from build123d import *

# Parameters (mm, degrees)
SALIENTE_EXTRUIR1_DEPTH = 55
CORTAR_EXTRUIR3_DEPTH   = 113.026782512
CORTAR_EXTRUIR4_DEPTH   = 116
CROQUIS6_R              = 1.6
CORTAR_EXTRUIR5_DEPTH   = 20
CORTAR_EXTRUIR6_START   = -10
CORTAR_EXTRUIR6_DEPTH   = 3
CROQUIS8_R              = 2.1
CORTAR_EXTRUIR8_DEPTH   = 116
MATRIZL1_COUNT          = 8
MATRIZL1_PITCH          = 10
CHAFL_N1_SIZE           = 1
CROQUIS9_R              = 2.1
CORTAR_EXTRUIR11_DEPTH  = 130.421791055
MATRIZL2_COUNT          = 6
MATRIZL2_PITCH          = 10


with BuildPart() as part:
    # Croquis1 → Saliente-Extruir1 (new body)
    with BuildSketch(Plane.XY):
        Polygon((15, -6.213203436), (15, 6.213203436), (6.213203436, 15), (-6.213203436, 15), (-15, 6.213203436), (-15, -6.213203436), (-6.213203436, -15), (6.213203436, -15), align=None)
    saliente_extruir1 = extrude(amount=SALIENTE_EXTRUIR1_DEPTH)

    # Simetría1: Saliente-Extruir1 across plane
    add(saliente_extruir1.mirror(Plane.XY.offset(55)))

    # Croquis4 → Cortar-Extruir3 (cut, through all)
    with BuildSketch(Plane(origin=(0, 0, 0), x_dir=(-1, 0, 0), z_dir=(0, 0, -1))):
        Polygon((-5.773502692, 0), (-2.886751346, -5), (2.886751346, -5), (5.773502692, 0), (2.886751346, 5), (-2.886751346, 5), align=None)
    extrude(amount=-CORTAR_EXTRUIR3_DEPTH, mode=Mode.SUBTRACT)

    # Croquis5 → Cortar-Extruir4 (cut, through all)
    with BuildSketch(Plane.XZ.offset(15)):
        Polygon((-6.213203436, 110), (-6.213203436, 78.298736304), (-15, 40.569524353), (-15, 110), align=None)
    extrude(amount=-CORTAR_EXTRUIR4_DEPTH, mode=Mode.SUBTRACT)

    # Croquis6 → Cortar-Extruir5 (cut)
    with BuildSketch(Plane.XY.offset(110)):
        with Locations((0, 11)):
            Circle(CROQUIS6_R)
        with Locations((7.778174593, 7.778174593)):
            Circle(CROQUIS6_R)
        with Locations((11, 0)):
            Circle(CROQUIS6_R)
        with Locations((7.778174593, -7.778174593)):
            Circle(CROQUIS6_R)
        with Locations((0, -11)):
            Circle(CROQUIS6_R)
    extrude(amount=-CORTAR_EXTRUIR5_DEPTH, mode=Mode.SUBTRACT)

    # Croquis7 → Cortar-Extruir6 (cut)
    with BuildSketch(Plane.XY.offset(110).offset(CORTAR_EXTRUIR6_START)):
        Polygon((-2.75, 12.58771324), (-2.75, 18.463203436), (2.75, 23.963203436), (2.75, 12.58771324), (2.75, 9.41228676), (0, 7.824573519), (-2.75, 9.41228676), align=None)
        Polygon((6.956313744, 10.84540104), (11.110912703, 15), (18.889087297, 15), (10.84540104, 6.956313744), (8.600035443, 4.710948146), (5.532808996, 5.532808996), (4.710948146, 8.600035443), align=None)
        Polygon((12.58771324, 2.75), (18.463203436, 2.75), (23.963203436, -2.75), (12.58771324, -2.75), (9.41228676, -2.75), (7.824573519, 0), (9.41228676, 2.75), align=None)
        Polygon((10.84540104, -6.956313744), (15, -11.110912703), (15, -18.889087297), (6.956313744, -10.84540104), (4.710948146, -8.600035443), (5.532808996, -5.532808996), (8.600035443, -4.710948146), align=None)
        Polygon((2.75, -12.58771324), (2.75, -18.463203436), (-2.75, -23.963203436), (-2.75, -12.58771324), (-2.75, -9.41228676), (0, -7.824573519), (2.75, -9.41228676), align=None)
    extrude(amount=-CORTAR_EXTRUIR6_DEPTH, mode=Mode.SUBTRACT)

    # Croquis8 → Cortar-Extruir8 (cut, through all)
    with BuildSketch(Plane.XZ.offset(15)):
        with Locations((0, 5)):
            Circle(CROQUIS8_R)
    cortar_extruir8 = extrude(amount=-CORTAR_EXTRUIR8_DEPTH, mode=Mode.SUBTRACT)

    # MatrizL1: Cortar-Extruir8 ×8
    with Locations(*[(0, 0, i * MATRIZL1_PITCH) for i in range(1, MATRIZL1_COUNT)]):
        add(cortar_extruir8, mode=Mode.SUBTRACT)

    # Chaflán1
    # the kernel refuses this chamfer: 1 mm, written as the material it takes off along each edge
    with BuildSketch(Plane(origin=(-6.213203436, -15, 112.571682988), x_dir=(0.9996219169112968, -0.027495876610585623, 0), z_dir=(0, 0, -1))) as chafl_n1_piece_1_section:
        Polygon((CHAFL_N1_SIZE * 0.999621916911, -CHAFL_N1_SIZE * 0.0274958766106), (-CHAFL_N1_SIZE * 0.0274958766106, -CHAFL_N1_SIZE * 0.999621916911), (0, 0), align=None)
    chafl_n1_piece_1 = extrude(amount=34.272946684, mode=Mode.PRIVATE)
    chafl_n1_piece_1 = split(chafl_n1_piece_1, bisect_by=Plane(origin=(-2.540552648, -14.662726337, 94.068558556), z_dir=(-0.9739364396780411, 0, 0.22682110013678505)), keep=Keep.TOP, mode=Mode.PRIVATE)
    add(chafl_n1_piece_1, mode=Mode.SUBTRACT)
    with BuildSketch(Plane(origin=(-6.213203436, 15, 78.298736304), x_dir=(-0.027495876610583055, -0.9996219169112968, 0), z_dir=(0, 0, 1))) as chafl_n1_piece_2_section:
        Polygon((CHAFL_N1_SIZE * 0.999621916911, CHAFL_N1_SIZE * 0.0274958766106), (-CHAFL_N1_SIZE * 0.0274958766106, CHAFL_N1_SIZE * 0.999621916911), (0, 0), align=None)
    chafl_n1_piece_2 = extrude(amount=34.272946684, mode=Mode.PRIVATE)
    chafl_n1_piece_2 = split(chafl_n1_piece_2, bisect_by=Plane(origin=(-2.540552648, 14.662726337, 94.068558556), z_dir=(-0.9739364396780411, 0, 0.22682110013678505)), keep=Keep.TOP, mode=Mode.PRIVATE)
    add(chafl_n1_piece_2, mode=Mode.SUBTRACT)
    with BuildSketch(Plane(origin=(-6.213203436, -17.571682988, 110), x_dir=(0.999621916911297, 0, 0.027495876610582174), z_dir=(0, 1, 0))) as chafl_n1_piece_3:
        Polygon((CHAFL_N1_SIZE * 0.999621916911, CHAFL_N1_SIZE * 0.0274958766106), (-CHAFL_N1_SIZE * 0.0274958766106, CHAFL_N1_SIZE * 0.999621916911), (0, 0), align=None)
    extrude(amount=35.143365976, mode=Mode.SUBTRACT)

    # Croquis9 → Cortar-Extruir11 (cut, through all)
    with BuildSketch(Plane(origin=(15, 0, -15), x_dir=(0, 0, -1), z_dir=(-1, 0, 0))):
        with Locations((-25, 0)):
            Circle(CROQUIS9_R)
    cortar_extruir11 = extrude(amount=CORTAR_EXTRUIR11_DEPTH, mode=Mode.SUBTRACT)

    # MatrizL2: Cortar-Extruir11 ×6
    with Locations(*[(0, 0, i * MATRIZL2_PITCH) for i in range(1, MATRIZL2_COUNT)]):
        add(cortar_extruir11, mode=Mode.SUBTRACT)


solid = part.part
Build history of the part. All positions in model axes, mm. A direction names the side the tool comes from. Coordinates: 2 decimals unless noted, no trailing zeros. Order: outer loops, then holes, each group sorted by start corner. A loop starts at its lowest first (then second) coordinate and runs counter-clockwise, first axis right, second up. Notation, with made-up numbers: (81, 61.25) - (105, 61.25) arc R21 ccw to (105, 78.25) - close; hole circle Ø2 at (16.5, 59.25). An arc over 180 degrees is marked (long way). Put each result on its own line as item: value.
1. Tool access for faces 5 (the face through (13, 0, 100)), 6 (the face through (7.57, 9.365, 93.549)), 7 (the face through (-2.75, 12, 99)), 8 (the face through (0, -13, 97)), 9 (the face through (7.04, -5.13, 98.52)): list every direction of +Z, -Z, +X, -X, +Y, -Y with a clear straight run to the whole face (end or side of a thin tool).
Answer sheet:
face 5: +X
face 6: +Z
face 7: +Y
face 8: -Y
face 9: none
2. Pull direction Z, two halves, no side cores. Call faces 1 (the face through (-6.213, 0, 94)), 2 (the face through (10, 9, 97)), 3 (the face through (8.63, -1.394, 98.521)), 4 (the face through (7, 0, 110)): pulls with the +Z half, pulls with the -Z half, needs draft (parallel to the pull), parting line crosses it, or undercut.
Answer sheet:
face 1: needs draft
face 2: undercut
face 3: undercut
face 4: pulls with the +Z half
3. Saw through at A-A (z = 35). Write the cut outline in (x, y).
Answer sheet:
outline: (-15, -6.21) - (-6.21, -15) - (-2.1, -15) - (-2.1, -5) - (-2.89, -5) - (-5.77, 0) - (-2.89, 5) - (-2.1, 5) - (-2.1, 15) - (-6.21, 15) - (-15, 6.21) - close; (2.1, -15) - (6.21, -15) - (15, -6.21) - (15, 6.21) - (6.21, 15) - (2.1, 15) - (2.1, 5) - (2.89, 5) - (5.77, 0) - (2.89, -5) - (2.1, -5) - close
4. Saw through at B-B (z = 10). Write the cut outline in (x, y), and give its area (3 significant figures).
Answer sheet:
outline: (-15, -6.21) - (-6.21, -15) - (6.21, -15) - (15, -6.21) - (15, -2.1) - (4.56, -2.1) - (2.89, -5) - (-2.89, -5) - (-4.56, -2.1) - (-15, -2.1) - close; (-15, 2.1) - (-4.56, 2.1) - (-2.89, 5) - (2.89, 5) - (4.56, 2.1) - (15, 2.1) - (15, 6.21) - (6.21, 15) - (-6.21, 15) - (-15, 6.21) - close
area: 576 mm^2
5. Probe line 1 along Y through (x, z) = (1.75, 66.5); line 2 along X through (y, z) = (-3.5, 70.5); line 3 along Y through (x, z) = (8.75, 90.5). List the from-to ranges inside material, lowest first. Write a range as [from, to].
Answer sheet:
line 1: y = [-15, -5], [5, 15]
line 2: x = [-8.03, -3.75], [3.75, 15]
line 3: y = [-12.46, -9.05], [-6.51, 6.51], [9.05, 12.46]
6. Saw through at C-C (z = 55). Write the cut outline in (x, y).
Answer sheet:
outline: (-11.64, -9.57) - (-6.21, -15) - (-2.1, -15) - (-2.1, -5) - (-2.89, -5) - (-5.77, 0) - (-2.89, 5) - (-2.1, 5) - (-2.1, 15) - (-6.21, 15) - (-11.64, 9.57) - close; (2.1, -15) - (6.21, -15) - (15, -6.21) - (15, 6.21) - (6.21, 15) - (2.1, 15) - (2.1, 5) - (2.89, 5) - (5.77, 0) - (2.89, -5) - (2.1, -5) - close
7. Drop flat-ended pins along their axis: P1, Ø2.5, axis at x = 0, y = 11, coming from the -Z side; P2, Ø5, axis at x = -12, z = 38.5, coming from the -Y side; P3, Ø2.5, axis at y = -11, z = 98, coming from the -X side; P4, Ø1.5, axis at y = 11, z = 98, coming from the +X side. Give the stop position or say it passes through.
Answer sheet:
P1: stops at z = 0
P2: stops at y = -11.71
P3: stops at x = -6.21
P4: stops at x = 7.86
